```python
from build123d import *

# Parameters (mm, degrees)
CROQUIS1_W                                           = 42
CROQUIS1_H                                           = 42
SALIENTE_EXTRUIR1_DEPTH                              = 34
REDONDEO1_R                                          = 5
VACIADO1_T                                           = -2.1
CORTAR_EXTRUIR1_DEPTH                                = 59.974621346
CORTAR_EXTRUIR2_REACH                                = 62.087
CROQUIS4_W                                           = 13
CROQUIS4_H                                           = 15
REDONDEO2_R                                          = 5
REDONDEO3_R                                          = 1
REDONDEO4_R                                          = 0.25
CROQUIS5_R                                           = 3.65
SALIENTE_EXTRUIR2_DEPTH                              = 31.9
REFRENTADO_PARA_TORNILLO_TAP_N_CON_CABEZ_D           = 3.3
REFRENTADO_PARA_TORNILLO_TAP_N_CON_CABEZ_CSINK_D     = 6.72
REFRENTADO_PARA_TORNILLO_TAP_N_CON_CABEZ_CSINK_ANGLE = 90
CROQUIS16_R                                          = 1.3
SALIENTE_EXTRUIR3_DEPTH                              = 10


with BuildPart() as part:
    # Croquis1 → Saliente-Extruir1 (new body)
    with BuildSketch(Plane.XY):
        with Locations((2.622149837, 5.276923077)):
            Rectangle(CROQUIS1_W, CROQUIS1_H)
    extrude(amount=-SALIENTE_EXTRUIR1_DEPTH)

    # Redondeo1
    redondeo1_edges = [part.edges().sort_by_distance(p)[0] for p in [
        (-18.377850163, 26.276923077, -17),
        (23.622149837, 26.276923077, -17),
        (23.622149837, -15.723076923, -17),
        (-18.377850163, -15.723076923, -17),
    ]]
    fillet(redondeo1_edges, radius=REDONDEO1_R)

    # Vaciado1
    vaciado1_openings = [part.faces().sort_by_distance(p)[0] for p in [
        (2.622149837, 5.276923077, -34),
    ]]
    offset(amount=VACIADO1_T, openings=vaciado1_openings, kind=Kind.INTERSECTION)

    # Croquis2 → Cortar-Extruir1 (cut, through all)
    with BuildSketch(Plane(origin=(0, 26.276923077, 0), x_dir=(1, 0, 0), z_dir=(0, 1, 0))):
        Polygon((-11.557850163, 34), (16.792149837, 34), (16.792149837, 5), (11.442149837, 5), (11.442149837, 2.1), (-6.207850163, 2.1), (-6.207850163, 5), (-11.557850163, 5), align=None)
    extrude(amount=-CORTAR_EXTRUIR1_DEPTH, mode=Mode.SUBTRACT)

    # Croquis4 → Cortar-Extruir2 (cut, up to next)
    with BuildSketch(Plane(origin=(23.622149837, 0, 0), x_dir=(0, 0, -1), z_dir=(1, 0, 0)), mode=Mode.PRIVATE) as cortar_extruir2_sk1:
        with Locations((27.5, 5.276923077)):
            Rectangle(CROQUIS4_W, CROQUIS4_H)
    cortar_extruir2_tool1 = extrude(cortar_extruir2_sk1.sketch, amount=-CORTAR_EXTRUIR2_REACH, mode=Mode.PRIVATE) & part.part
    add(cortar_extruir2_tool1.solids().sort_by_distance((23.62215, 5.276923, -27.5))[0], mode=Mode.SUBTRACT)

    # Redondeo2
    redondeo2_edges = [part.edges().sort_by_distance(p)[0] for p in [
        (22.572149837, 12.776923077, -21),
        (22.572149837, -2.223076923, -21),
        (22.572149837, -2.223076923, -34),
        (22.572149837, 12.776923077, -34),
    ]]
    fillet(redondeo2_edges, radius=REDONDEO2_R)

    # Redondeo3
    redondeo3_edges = [part.edges().sort_by_distance(p)[0] for p in [
        (-11.557850163, 25.226923077, -5),
        (-11.557850163, -14.673076923, -5),
        (-11.557850163, 25.226923077, -34),
        (-11.557850163, -14.673076923, -34),
        (16.792149837, 25.226923077, -34),
        (16.792149837, -14.673076923, -34),
        (16.792149837, 25.226923077, -5),
        (16.792149837, -14.673076923, -5),
        (11.442149837, 25.226923077, -2.1),
        (11.442149837, -14.673076923, -2.1),
        (-6.207850163, 25.226923077, -5),
        (-6.207850163, -14.673076923, -5),
        (11.442149837, 25.226923077, -5),
        (11.442149837, -14.673076923, -5),
        (-6.207850163, 25.226923077, -2.1),
        (-6.207850163, -14.673076923, -2.1),
    ]]
    fillet(redondeo3_edges, radius=REDONDEO3_R)

    # Redondeo4
    redondeo4_edges = [part.edges().sort_by_distance(p)[0] for p in [
        (2.622149837, -15.723076923, 0),
        (-18.377850163, 5.276923077, 0),
        (23.622149837, 5.276923077, 0),
        (2.622149837, 26.276923077, 0),
        (22.157683743, 24.812456983, 0),
        (-16.913384069, 24.812456983, 0),
        (-16.913384069, -14.258610829, 0),
        (22.157683743, -14.258610829, 0),
    ]]
    fillet(redondeo4_edges, radius=REDONDEO4_R)

    # Croquis5 → Saliente-Extruir2 (add)
    with BuildSketch(Plane(origin=(0, 0, -2.1), x_dir=(-1, 0, 0), z_dir=(0, 0, -1))):
        with Locations((-18.122149837, 20.776923077)):
            Circle(CROQUIS5_R)
        with Locations((12.877850163, 20.776923077)):
            Circle(CROQUIS5_R)
        with Locations((-18.122149837, -10.223076923)):
            Circle(CROQUIS5_R)
        with Locations((12.877850163, -10.223076923)):
            Circle(CROQUIS5_R)
    extrude(amount=SALIENTE_EXTRUIR2_DEPTH)

    # Refrentado para tornillo tapón con cabeza plana de clavija de M31 (through all)
    with Locations(Plane.XY):
        with Locations((-12.877850163, 20.776923077), (-12.877850163, -10.223076923), (18.122149837, -10.223076923), (18.122149837, 20.776923077)):
            CounterSinkHole(REFRENTADO_PARA_TORNILLO_TAP_N_CON_CABEZ_D / 2, REFRENTADO_PARA_TORNILLO_TAP_N_CON_CABEZ_CSINK_D / 2, counter_sink_angle=REFRENTADO_PARA_TORNILLO_TAP_N_CON_CABEZ_CSINK_ANGLE)

    # Croquis16 → Saliente-Extruir3 (add)
    # profile 1 of 2: a face of its own
    with BuildSketch(Plane(origin=(0, 0, -2.1), x_dir=(-1, 0, 0), z_dir=(0, 0, -1))):
        with BuildLine():
            Line((-8.301696367, 14.817459435), (-8.301696367, 8.603842264))
            ThreePointArc((-8.301696367, 8.603842264), (-13.72041581, 11.71065085), (-8.301696367, 14.817459435))
        make_face()
        with Locations((-10.12041581, 11.71065085)):
            Circle(CROQUIS16_R, mode=Mode.SUBTRACT)
    # profile 2 of 2: a face of its own
    with BuildSketch(Plane(origin=(0, 0, -2.1), x_dir=(-1, 0, 0), z_dir=(0, 0, -1))):
        with BuildLine():
            Line((3.060124976, 14.818812033), (3.061604408, 8.605195038))
            ThreePointArc((3.061604408, 8.605195038), (8.479583981, 11.713293707), (3.060124976, 14.818812033))
        make_face()
        with Locations(Location((4.879584083, 11.712436564, 0), (0, 0, 180))):
            Circle(CROQUIS16_R, mode=Mode.SUBTRACT)
    extrude(amount=SALIENTE_EXTRUIR3_DEPTH)


solid = part.part
```
CAD build for the part. Positions are in the model's coordinates, mm. A direction names the side the tool comes from. Coordinates: 2 decimals unless noted, no trailing zeros. Write each loop counter-clockwise with the first axis right and the second up, starting at its lowest first coordinate (ties: lowest second). Pieces come first, ordered by that corner, then holes. Notation, with made-up numbers: (12.5, 88) -> (22.5, 88) arc R34 ccw to (22.5, 119) -> close; hole circle Ø11 at (51, -10.75). An arc over 180 degrees is marked (long way). Return JSON: item names as keys, results as strings. Group by question number.
Q1. Pull direction X, two halves, no side cores. Call faces 6 (the face through (-18.378, 5, -17)), 7 (the face through (23, -2.223, -27)), 8 (the face through (16.62, 17.45, -17.83)), 9 (the face through (22.119, -14.297, -17.361)): released by +X, released by -X, zero draft, split by the parting line, or undercut.
Q2. Which spindle directions (+Z, -Z, +X, -X, +Y, -Y) get a long thin tool onto all of the face, cutting with end or side? Do faces 1 (the face through (22.557, -3.727, -32.574)), 2 (the face through (-11.558, 25, -19)), 3 (the face through (-16.952, 24.773, -17.361)), 4 (the face through (3, 6, -2.1)), 5 (the face through (20, 22, -34)). Say none if no direction does.
Q3. Cut at A-A, the plane z = -25. State how many separate pieces and enclosed holes the cut face has, then the cut area to 3 significant figures.
Q4. Cut at B-B, the plane y = 3.5. Give the cut face in (x, z), then the cut area to 3 significant figures.
Q5. Drill centre lines: line 1 (X direction, y = 14.5, z = -24); line 2 (X direction, y = 19, z = -13); line 3 (X direction, y = -11, z = -7.5). Where is each one in solid material? Low to high.
Q6. Cut at D-D, the plane x = 0. Give the cut face in (y, z), then the cut area to 3 significant figures.
Q7. Flat gauge pins, fed straight in: pin 1 (6 mm diameter, centred on x = -5, y = 10.5, fed in from -Z); pin 2 (0.7 mm diameter, centred on y = 25, z = -3.5, fed in from -X); pin 3 (0.6 mm diameter, centred on y = -15, z = -19, fed in from +X). Where does each tip first touch, or does it go through?
Returned:
{
 "1": {"face 6": "released by -X", "face 7": "zero draft", "face 8": "undercut", "face 9": "released by +X"},
 "2": {"face 1": "-Z, +X", "face 2": "-Z, +Y", "face 3": "+Z, -Z, -X, +Y", "face 4": "-Z", "face 5": "-Z, +X, -X, +Y, -Y"},
 "3": {"separate pieces": "3", "enclosed holes": "4", "area": "299 mm2"},
 "4": {"outline": "(-18.38, -34) -> (-16.28, -34) -> (-16.28, -2.1) -> (21.52, -2.1) -> (21.52, -21) -> (23.62, -21) -> (23.62, -0.25) arc R0.25 ccw to (23.37, 0) -> (-18.13, 0) arc R0.25 ccw to (-18.38, -0.25) -> close", "area": "195 mm2"},
 "5": {"line 1": "x = -18.38 to -16.28, 21.52 to 23.62", "line 2": "x = -18.38 to -16.28, -16.07 to -9.69, 14.93 to 21.31, 21.52 to 23.62", "line 3": "x = -18.37 to -14.33, -11.42 to -9.31, 14.56 to 16.67, 19.58 to 23.61"},
 "6": {"outline": "(-15.72, -2.1) -> (26.28, -2.1) -> (26.28, -0.25) arc R0.25 ccw to (26.03, 0) -> (-15.47, 0) arc R0.25 ccw to (-15.72, -0.25) -> close", "area": "88.2 mm2"},
 "7": {"pin 1": "stops at z = -12.1", "pin 2": "stops at x = -17.07", "pin 3": "stops at x = 21.65"}
}
